Design review of the part built by this model. Coordinates are the model's own, in mm. A direction names the side the tool comes from. Round coordinates to 2 decimals unless told otherwise and drop trailing zeros. Order: outer loops, then holes, each group sorted by start corner. A loop starts at its lowest first (then second) coordinate and runs counter-clockwise, first axis right, second up. Notation, with made-up numbers: (36, 59) - (81, 59) arc R14 ccw to (81, 68) - close; hole circle Ø4 at (39.25, 39). An arc over 180 degrees is marked (long way). Answer as a JSON object with one key per item and string values. Group by question number.
from build123d import *

# Parameters (mm, degrees)
F0_R     = 4
F0_R_2   = 1.75
F1_DEPTH = 1.75
F2_DEPTH = 4.5
F3_R     = 1.5
F4_DEPTH = 5


with BuildPart() as f1:
    # F0 (on Top) → F1 (new body, symmetric)
    with BuildSketch(Plane.XY):
        Circle(F0_R)
        Circle(F0_R_2, mode=Mode.SUBTRACT)
    extrude(amount=F1_DEPTH, both=True)

    # F0 (on Top) → F2 (join, symmetric)
    with BuildSketch(Plane.XY):
        Circle(F0_R_2)
    extrude(amount=F2_DEPTH, both=True)

    # F3 (on Right) → F4 (cut, symmetric)
    with BuildSketch(Plane.YZ):
        Circle(F3_R)
    extrude(amount=F4_DEPTH, both=True, mode=Mode.SUBTRACT)


solid = f1.part
1. Tool access review of faces 1 (the cylindrical face through (1.617, -0.67, 3.144)), 2 (the flat face through (0, 0, -4.5)), 3 (the flat face through (2, -1, -1.75)): name each direction out of +Z, -Z, +X, -X, +Y, -Y from which nothing blocks a thin tool from reaching the whole face with its end or side.
2. Take a section at C-C, the plane z = 0. Give the boundary of the cut face in (x, y), then the cut area to 3 significant figures.
3. Take a section at B-B, the plane x = 0. Give the boundary of the cut face in (y, z).
4. Take a section at A-A, the plane y = 0. Give the boundary of the cut face in (x, z).
5. Take a section at D-D, the plane y = 1. Give the boundary of the cut face in (x, z).
6. To check wall thickness, follow line 1 (Z direction, x = 0, y = 0); line 2 (Z direction, x = 2.25, y = 0); line 3 (Y direction, x = 0, z = 0). State the ranges of each line that lie inside material, in increasing order. Write a range as from..to.
7. Clearance check with flat-ended pins moving along their axes: P1, Ø4, axis at x = -2, y = 2, coming from the -Z side; P2, Ø2, axis at y = -1.5, z = 3, coming from the -X side; P3, Ø1.5, axis at y = -2.5, z = -2, coming from the -X side; P4, Ø1.5, axis at x = -2.5, z = 0, coming from the +Y side. State where each tip first meets the part, or that it passes through.
8. Mouldability with a two-part tool opening along Y and no side actions: class faces 4 (the cylindrical face through (1.617, -0.67, -3.106)), 5 (the cylindrical face through (0.06, -1.5, 0.07)), 6 (the flat face through (2, -1, 1.75)) as pulls with the +Y half, pulls with the -Y half, needs draft (parallel to the pull), parting line crosses it, or undercut.
Response values:
{
 "1": {"face 1": "+Z", "face 2": "-Z, +X, -X, +Y, -Y", "face 3": "-Z"},
 "2": {"outline": "(-3.71, -1.5) arc R4 ccw to (3.71, -1.5) - close; (-3.71, 1.5) - (3.71, 1.5) arc R4 ccw to start", "area": "26.8 mm2"},
 "3": {"outline": "(-4, -1.75) - (-1.75, -1.75) - (-1.75, -4.5) - (1.75, -4.5) - (1.75, -1.75) - (4, -1.75) - (4, 1.75) - (1.75, 1.75) - (1.75, 4.5) - (-1.75, 4.5) - (-1.75, 1.75) - (-4, 1.75) - close; hole circle Ø3 at (0, 0)"},
 "4": {"outline": "(-4, -1.75) - (-1.75, -1.75) - (-1.75, -4.5) - (1.75, -4.5) - (1.75, -1.75) - (4, -1.75) - (4, -1.5) - (-4, -1.5) - close; (-4, 1.5) - (4, 1.5) - (4, 1.75) - (1.75, 1.75) - (1.75, 4.5) - (-1.75, 4.5) - (-1.75, 1.75) - (-4, 1.75) - close"},
 "5": {"outline": "(-3.87, -1.75) - (-1.44, -1.75) - (-1.44, -4.5) - (1.44, -4.5) - (1.44, -1.75) - (3.87, -1.75) - (3.87, -1.12) - (-3.87, -1.12) - close; (-3.87, 1.12) - (3.87, 1.12) - (3.87, 1.75) - (1.44, 1.75) - (1.44, 4.5) - (-1.44, 4.5) - (-1.44, 1.75) - (-3.87, 1.75) - close"},
 "6": {"line 1": "-4.5..-1.5, 1.5..4.5", "line 2": "-1.75..-1.5, 1.5..1.75", "line 3": "-4..-1.5, 1.5..4"},
 "7": {"P1": "z = -4.5", "P2": "x = -1.68", "P3": "x = -3.58", "P4": "y = 3.6"},
 "8": {"face 4": "parting line crosses it", "face 5": "undercut", "face 6": "needs draft"}
}
